For this review, use the dimensioned drawing (mm, ordinates from the lowest corner) and the shaded views. A direction names the side the tool comes from. Coordinates: 2 decimals unless noted, no trailing zeros. Order: outer loops, then holes, each group sorted by start corner. A loop starts at its lowest first (then second) coordinate and runs counter-clockwise, first axis right, second up. Notation, with made-up numbers: (-0.75, 21.25) -> (34.25, 21.25) arc R23 ccw to (34.25, 58.25) -> close; hole circle Ø6 at (69, 74.5). An arc over 180 degrees is marked (long way). Use CSV: the item, a comma, the result in double quotes. Start each with the question number.
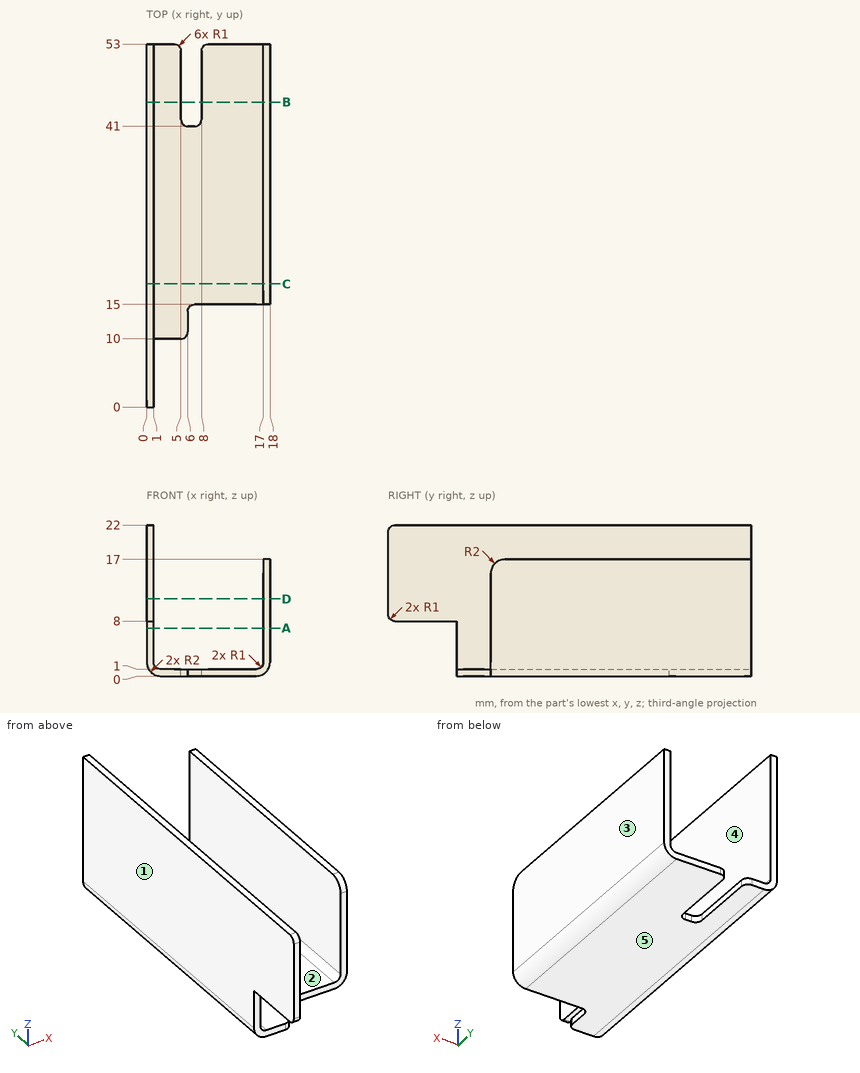
Q1. Add section D-D, the plane z = 11.25. State the section outline as (x, y) points.
Q2. Draft analysis for pull direction X (two halves, no side actions). For the marked faces 3, 4 and 5, state which applies: +X half, -X half, draft (parallel to the pull), parting line (faces both ways), or undercut.
Q3. Add section B-B, the plane y = 44.5. State the section outline as (x, z) points.
Q4. For the marked faces 1 and 2, list the 3-axis set-ups (+Z, -Z, +X, -X, +Y, -Y) from which the entire face can be reached by the end or side of a thin tool; tool diameter is ignored.
Q5. Add section C-C, the plane y = 18. State the section outline as (x, z) points, then the cut area to 3 significant figures.
Q6. Add section A-A, the plane z = 7. State the section outline as (x, y) points, then the cut area to 3 significant figures.
Q7. Clearance check with flat-ended pins moving along their axes: pin 1 Ø2 at (x, y) = (8.5, 18) entering from +Z; pin 2 Ø0.5 at (x, y) = (17.5, 26.5) entering from +Z; pin 3 Ø0.8 at (x, z) = (6.5, 0.5) entering from +Y. State where each tip first meets the part, or that it passes through.
Q8. To check wall thickness, follow probe 1 along X at (y, z) = (30.5, 12); probe 2 along Z at (x, y) = (14, 28.5). State the ranges of each line that lie inside material, in increasing order.
Answer block:
1,outline,"(0, 0) -> (1, 0) -> (1, 53) -> (0, 53) -> close; (17, 15) -> (18, 15) -> (18, 53) -> (17, 53) -> close"
2,face 3,"+X half"
2,face 4,"undercut"
2,face 5,"draft"
3,outline,"(0, 2) arc R2 ccw to (2, 0) -> (5, 0) -> (5, 1) -> (2, 1) arc R1 cw to (1, 2) -> (1, 22) -> (0, 22) -> close; (8, 0) -> (16, 0) arc R2 ccw to (18, 2) -> (18, 17) -> (17, 17) -> (17, 2) arc R1 cw to (16, 1) -> (8, 1) -> close"
4,face 1,"+Z, -Z, -X, +Y, -Y"
4,face 2,"+Z, +Y, -Y"
5,outline,"(0, 2) arc R2 ccw to (2, 0) -> (16, 0) arc R2 ccw to (18, 2) -> (18, 17) -> (17, 17) -> (17, 2) arc R1 cw to (16, 1) -> (2, 1) arc R1 cw to (1, 2) -> (1, 22) -> (0, 22) -> close"
5,area,"53.7 mm²"
6,outline,"(0, 10) -> (1, 10) -> (1, 53) -> (0, 53) -> close; (17, 15) -> (18, 15) -> (18, 53) -> (17, 53) -> close"
6,area,"81.0 mm²"
7,pin 1,"stops at z = 1"
7,pin 2,"stops at z = 17"
7,pin 3,"stops at y = 41"
8,probe 1,"x = 0 to 1, 17 to 18"
8,probe 2,"z = 0 to 1"
